from build123d import *

# Parameters (mm, degrees)
F0_R     = 2.38125
F1_DEPTH = 3.175
F2_SIZE  = 3.175


with BuildPart() as f1:
    # F0 (on Front) → F1 (new body, symmetric)
    with BuildSketch(Plane.XZ):
        with BuildLine():
            Line((57.15, 63.5), (-57.15, 63.5))
            ThreePointArc((-57.15, 63.5), (-61.640128, 61.640128), (-63.5, 57.15))
            Line((-63.5, 57.15), (-63.5, -57.15))
            ThreePointArc((-63.5, -57.15), (-61.640128, -61.640128), (-57.15, -63.5))
            Line((-57.15, -63.5), (57.15, -63.5))
            ThreePointArc((57.15, -63.5), (61.640128, -61.640128), (63.5, -57.15))
            Line((63.5, -57.15), (63.5, 57.15))
            ThreePointArc((63.5, 57.15), (61.640128, 61.640128), (57.15, 63.5))
        make_face()
        with Locations((-47.625, -47.625)):
            Circle(F0_R, mode=Mode.SUBTRACT)
        with Locations((47.625, -47.625)):
            Circle(F0_R, mode=Mode.SUBTRACT)
        with Locations((-47.625, 47.625)):
            Circle(F0_R, mode=Mode.SUBTRACT)
        with BuildLine():
            Line((-32.600739, -12.472045), (-5.499261, 34.469091))
            ThreePointArc((-5.499261, 34.469091), (0, 37.644091), (5.499261, 34.469091))
            Line((5.499261, 34.469091), (32.600739, -12.472045))
            ThreePointArc((32.600739, -12.472045), (32.600739, -18.822045), (27.101477, -21.997045))
            Line((27.101477, -21.997045), (-27.101477, -21.997045))
            ThreePointArc((-27.101477, -21.997045), (-32.600739, -18.822045), (-32.600739, -12.472045))
        make_face(mode=Mode.SUBTRACT)
        with Locations((47.625, 47.625)):
            Circle(F0_R, mode=Mode.SUBTRACT)
    extrude(amount=F1_DEPTH, both=True)

    # F2
    f2_edges = [f1.edges().sort_by_distance(p)[0] for p in [
        (-50.00625, -3.175, 47.625),
        (-50.00625, -3.175, -47.625),
        (45.24375, -3.175, -47.625),
        (45.24375, -3.175, 47.625),
    ]]
    chamfer(f2_edges, length=F2_SIZE)


solid = f1.part
Could you check a few things on this model? Use its own coordinates, in mm. A direction names the side the tool comes from. Round coordinates to 2 decimals unless told otherwise and drop trailing zeros. Write each loop counter-clockwise with the first axis right and the second up, starting at its lowest first coordinate (ties: lowest second). Pieces come first, ordered by that corner, then holes. Notation, with made-up numbers: (-15, -3.75) - (28, -3.75) arc R20 ccw to (28, 6.25) - close; hole circle Ø3 at (30, 76). An arc over 180 degrees is marked (long way). Put each result on its own line as item: value. Start each with the question number.
(1) For faces 1 (the cylindrical face through (-32.554, -0.044, -18.902)), 2 (the flat face through (1, 0, 63.5)), which set-ups out of +Z, -Z, +X, -X, +Y, -Y let a thin tool reach every point of the face, with its end or its side?
(2) I want a section at B-B, the plane x = 0. Please give me the cut outline in (y, z) (3 decimals).
(3) Will these pins go through, and if not, where does the flat tip stop? pin 1 (3 mm diameter, centred on x = -47.625, z = -47.625, fed in from -Y); pin 2 (6 mm diameter, centred on x = -47.625, z = 47.625, fed in from -Y).
(4) I want a section at C-C, the plane y = -2. Give the number of separate pieces and of enclosed holes in the cut face, plus the area to 3 significant figures.
(5) I need wall thicknesses on probe 1 along Z at (x, y) = (50, -0.5); probe 2 along Z at (x, y) = (-7.5, 0.25); probe 3 along X at (y, z) = (0.5, -46.5). Which ranges of each line are inside material? Lowest first, please.
(6) I want a section at A-A, the plane z = 30. Please give me the cut outline in (x, y) (1 decimal).
(7) Thinking about a two-plate mould opening in Z: for faces 3 (the flat face through (0, 0, -21.997)), 4 (the cylindrical face through (61.69, -0.04, 61.59)), 5 (the conical face through (45.092, -0.154, -47.514)), 6 (the flat face through (27, 3.175, 1)), which applies, released by +Z, released by -Z, zero draft, split by the parting line, or undercut?
Here are the results:
1. face 1: +Y, -Y
1. face 2: +Z, +X, -X, +Y, -Y
2. outline: (-3.175, -63.5) - (3.175, -63.5) - (3.175, -21.997) - (-3.175, -21.997) - close; (-3.175, 37.644) - (3.175, 37.644) - (3.175, 63.5) - (-3.175, 63.5) - close
3. pin 1: passes through
3. pin 2: stops at y = -0.62
4. separate pieces: 1
4. enclosed holes: 5
4. area: 13,400 mm^2
5. probe 1: z = -63.5 to -49.26, -45.99 to 45.99, 49.26 to 63.5
5. probe 2: z = -63.5 to -22, 31 to 63.5
5. probe 3: x = -63.5 to -49.72, -45.53 to 45.53, 49.72 to 63.5
6. outline: (-63.5, -3.2) - (-8.1, -3.2) - (-8.1, 3.2) - (-63.5, 3.2) - close; (8.1, -3.2) - (63.5, -3.2) - (63.5, 3.2) - (8.1, 3.2) - close
7. face 3: undercut
7. face 4: released by +Z
7. face 5: undercut
7. face 6: zero draft
